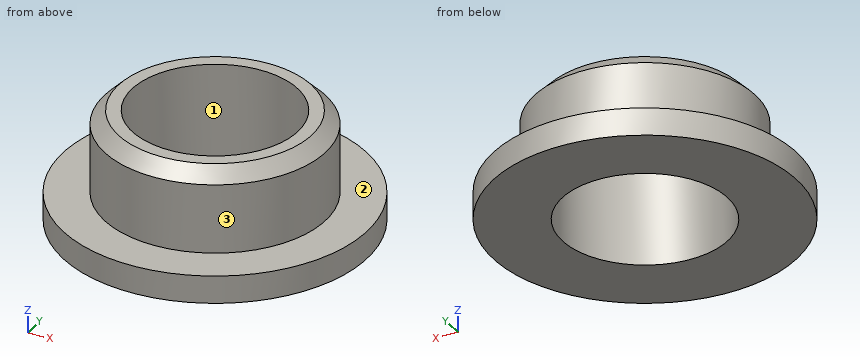
Autodesk Inventor part; units mm, degrees
ref_plane "YZ Plane" through (0, 0, 0) normal (1, 0, 0) x (0, 1, 0)
ref_plane "XZ Plane" through (0, 0, 0) normal (0, 1, 0) x (-1, 0, 0)
ref_plane "XY Plane" through (0, 0, 0) normal (0, 0, 1) x (1, 0, 0)
sketch "スケッチ1" plane through (0, 0, 0) normal (0, 0, 1) x (1, 0, 0)
  circle A0 centre (0, 0) radius 5.5
  circle A1 centre (0, 0) radius 3
  dimension "d0" = 11
  dimension "d1" = 6
extrude "押し出し1" add sketch "スケッチ1" along normal blind 1
sketch "スケッチ2" plane through (0, 0, 1) normal (0, 0, 1) x (1, 0, 0)
  circle A0 centre (0, 0) radius 4
  circle A1 centre (0, 0) radius 3
  dimension "d4" = 8
extrude "押し出し2" add sketch "スケッチ2" along normal blind 3
chamfer "面取り1" distance 0.5 angle 45 1 edges at (-4, 0, 4)
properties part number "オイレス6-10" material "アセタール樹脂、黒"
Check sheet for the modelled part. Datum: model origin and axes. Units: mm. Face numbers are marked on the shaded views. Round coordinates to 2 decimals unless told otherwise and drop trailing zeros. Order: outer loops, then holes, each group sorted by start corner. A loop starts at its lowest first (then second) coordinate and runs counter-clockwise, first axis right, second up. Notation, with made-up numbers: (-39, -24.75) -> (-27, -24.75) arc R32 cw to (-27, 6.25) -> close; hole circle Ø3 at (86.25, 40.25). An arc over 180 degrees is marked (long way). One line per item, written item: value. Start each with the question number.
Q1. Cross-section at D-D (y = 4.5). Record the boundary of the cut face in (x, z).
Q2. Thickness scan on line 1 (Y direction, x = 0, z = 2.45); line 2 (Z direction, x = -2.25, y = -4); line 3 (X direction, y = -0.25, z = 3.85). Record the ranges inside material, lowest first.
Q3. Gauge pin test, flat end, axial feed: pin 1 Ø2 at (y, z) = (1, 2.5) entering from -X. Record the tip position at first contact, or that the pin passes through.
Q4. Cross-section at A-A (x = 0). Record the boundary of the cut face in (y, z).
Q5. Cross-section at C-C (z = 2.4). Record the boundary of the cut face in (x, y).
Q6. Mould release check, pull along X, two halves, no side actions. Record for the marked faces 1, 2 and 3: pulls with the +X half, pulls with the -X half, needs draft (parallel to the pull), parting line crosses it, or undercut.
Completed:
1. outline: (-3.16, 0) -> (3.16, 0) -> (3.16, 1) -> (-3.16, 1) -> close
2. line 1: y = -4 to -3, 3 to 4
2. line 2: z = 0 to 1
2. line 3: x = -3.64 to -2.99, 2.99 to 3.64
3. pin 1: stops at x = -4
4. outline: (-5.5, 0) -> (-3, 0) -> (-3, 4) -> (-3.5, 4) -> (-4, 3.5) -> (-4, 1) -> (-5.5, 1) -> close; (3, 0) -> (5.5, 0) -> (5.5, 1) -> (4, 1) -> (4, 3.5) -> (3.5, 4) -> (3, 4) -> close
5. outline: circle Ø8 at (0, 0); hole circle Ø6 at (0, 0)
6. face 1: undercut
6. face 2: needs draft
6. face 3: parting line crosses it
